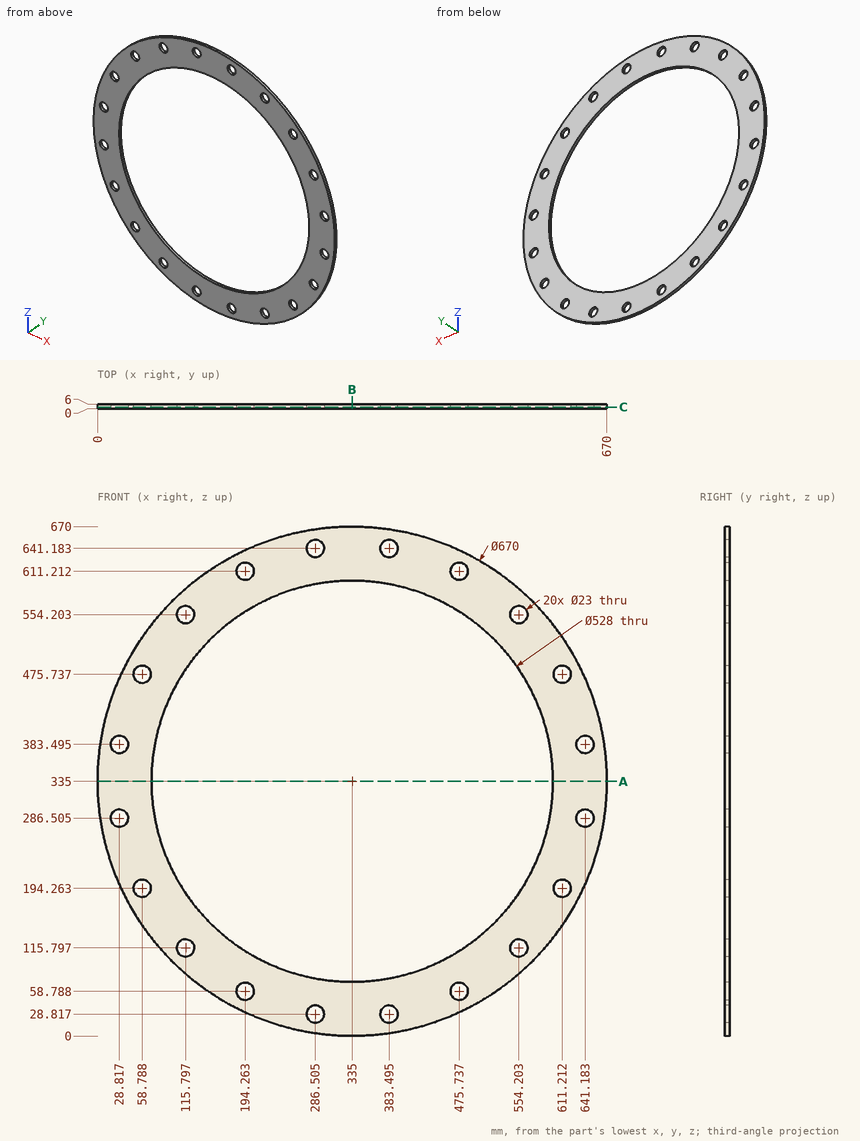
Verification items for this drawing (mm, ordinates from the low corner). Round coordinates to 2 decimals unless told otherwise and drop trailing zeros. Order: outer loops, then holes, each group sorted by start corner. A loop starts at its lowest first (then second) coordinate and runs counter-clockwise, first axis right, second up. Notation, with made-up numbers: M 18.5,-31.75 L 67.5,-31.75 A20 cw 67.5,-8.75 Z; hole C -6,-30.5 d6. An arc over 180 degrees is marked long. Answer in a Markdown table with one row per item. Add a question column.
Item 1: Depth check by flat-ended pin: pin 1 Ø1.5 at (x, y) = (253, 2.5) entering from +Z; pin 2 Ø14 at (x, z) = (115.8, 554.2) entering from +Y; pin 3 Ø1.5 at (y, z) = (0.5, 441.5) entering from -X; pin 4 Ø1.5 at (y, z) = (2.5, 601) entering from -X (1 decimal). Enter the tip coordinate at first touch or a pass-through.
Item 2: Sectioned sample at A-A, the plane z = 335. Enter the section's corners in (x, y).
Item 3: Sectioned sample at C-C, the plane y = 1.8. State how many separate pieces and enclosed holes the cut face has, plus the area to 3 significant figures.
Item 4: Material ranges on L1, parallel to X at y = 4.7, z = 640 (1 decimal); L2, parallel to X at y = 0.9, z = 38.5 (1 decimal); L3, parallel to X at y = 2.9, z = 547 (1 decimal), recorded low to high. Write a range as [from, to].
Item 5: Sectioned sample at B-B, the plane x = 335. Enter the section's corners in (y, z).
Filled in:
| question | item | result |
|---|---|---|
| 1 | pin 1 | stops at z = 660 |
| 1 | pin 2 | passes through |
| 1 | pin 3 | stops at x = 17.13 |
| 1 | pin 4 | stops at x = 130.4 |
| 2 | outline | M 0,0 L 71,0 L 71,6 L 0,6 Z; M 599,0 L 670,0 L 670,6 L 599,6 Z |
| 3 | separate pieces | 1 |
| 3 | enclosed holes | 21 |
| 3 | area | 125,000 mm² |
| 4 | L1 | x = [196.4, 275.1], [297.9, 372.1], [394.9, 473.6] |
| 4 | L2 | x = [179.1, 280.3], [292.7, 377.3], [389.7, 490.9] |
| 4 | L3 | x = [75.6, 106.8], [124.8, 177.7], [492.3, 545.2], [563.2, 594.4] |
| 5 | outline | M 0,0 L 6,0 L 6,71 L 0,71 Z; M 0,599 L 6,599 L 6,670 L 0,670 Z |
